CAD build for the part. Positions are in the model's coordinates, mm. A direction names the side the tool comes from. Round coordinates to 2 decimals unless told otherwise and drop trailing zeros. Write each loop counter-clockwise with the first axis right and the second up, starting at its lowest first coordinate (ties: lowest second). Pieces come first, ordered by that corner, then holes. Notation, with made-up numbers: (69, 35) - (95, 35) arc R20 ccw to (95, 65) - close; hole circle Ø2 at (-1, -36). An arc over 180 degrees is marked (long way). Use one line per item in the form item = value. Start each with the question number.
Item 1: Drill centre lines: L1, parallel to Z at x = -10.68, y = 13.55; L2, parallel to Y at x = 2, z = -3; L3, parallel to X at y = 9.5, z = 3.25. Where is each one in solid material? Low to high.
Item 2: Pull direction X, two halves, no side cores. Call faces 1 (the cylindrical face through (1.56, 7.23, 4.96)), 2 (the flat face through (6, 6, 0)), 3 (the flat face through (-1, 15.66, 0)): +X half, -X half, draft (parallel to the pull), parting line (faces both ways), or undercut.
Item 3: Tool access for faces 4 (the flat face through (0, 14.66, 0)), 5 (the flat face through (-2, 13, 7)), 6 (the flat face through (-4, 13, -7)), 7 (the cylindrical face through (-11.59, 13.05, -6.81)), 8 (the cylindrical face through (4.748, 15.098, 0.089)): list every direction of +Z, -Z, +X, -X, +Y, -Y with a clear straight run to the whole face (end or side of a thin tool).
Item 4: Pin check, flat tips, straight feed: pin 1 (4 mm diameter, centred on x = -8.5, z = -3.5, fed in from -Y); pin 2 (4 mm diameter, centred on x = -10.68, z = -8, fed in from +Y); pin 3 (4 mm diameter, centred on y = 5, z = -6, fed in from -X); pin 4 (2 mm diameter, centred on x = -7, y = 12, fed in from -Z). Stop position of each tip, or through.
Item 5: Band-saw the part on A-A, the plane z = -8. List the corners of the cut face in (x, y).
Item 6: Band-saw the part on D-D, the plane z = 8. List the corners of the cut face in (x, y).
Item 7: Band-saw the part on B-B, the plane x = -10.68. List the corners of the cut face in (y, z).
Item 8: Band-saw the part on C-C, the plane y = 1.75. List the corners of the cut face in (x, z).
from build123d import *
from build123d.topology import SkipClean

# Parameters (mm, degrees)
SKETCH1_R           = 7
SKETCH1_R_2         = 5.2
BOSS_EXTRUDE1_DEPTH = 15.66
BOSS_EXTRUDE2_START = -3.6
SKETCH2_W           = 6
SKETCH2_H           = 4
BOSS_EXTRUDE2_DEPTH = 3.6
CUT_EXTRUDE2_START  = -1.6
SKETCH2_3_W         = 6
SKETCH2_3_H         = 4
CUT_EXTRUDE2_DEPTH  = 1.6
SKETCH4_R           = 1.5
CUT_EXTRUDE1_DEPTH  = 10
FILLET7_R           = 3
BOSS_EXTRUDE3_START = -1
SKETCH5_R           = 5.2
BOSS_EXTRUDE3_DEPTH = 1
CUT_EXTRUDE3_DEPTH  = 15.66
FILLET8_R           = 3


with BuildPart() as part:
    # Sketch1 → Boss-Extrude1 (new body)
    with BuildSketch(Plane(origin=(0, 0, 0), x_dir=(1, 0, 0), z_dir=(0, 1, 0))):
        with Locations(Location((0, 0, 0), (0, 0, 270))):
            Circle(SKETCH1_R)
        with Locations(Location((0, 0, 0), (0, 0, 270))):
            Circle(SKETCH1_R_2, mode=Mode.SUBTRACT)
    extrude(amount=BOSS_EXTRUDE1_DEPTH)

    # Sketch2 → Boss-Extrude2 (add)
    with BuildSketch(Plane(origin=(0, 15.66, 0), x_dir=(1, 0, 0), z_dir=(0, 1, 0)).offset(BOSS_EXTRUDE2_START)):
        with Locations((-10.67, -9)):
            Rectangle(SKETCH2_W, SKETCH2_H)
        with BuildLine():
            ThreePointArc((0, -7), (-7, 0), (0, 7))
            Line((0, 7), (-7.67, 7))
            Line((-7.67, 7), (-13.67, 7))
            Line((-13.67, 7), (-13.67, -7))
            Line((-13.67, -7), (-7.67, -7))
            Line((-7.67, -7), (0, -7))
        make_face()
        with Locations((-10.67, 9)):
            Rectangle(SKETCH2_W, SKETCH2_H)
    extrude(amount=BOSS_EXTRUDE2_DEPTH)

    # Sketch2<3> → Cut-Extrude2 (cut)
    with SkipClean():  # the faces are left unmerged after this step: merging them gives an invalid solid
        with BuildSketch(Plane(origin=(0, 15.66, 0), x_dir=(1, 0, 0), z_dir=(0, 1, 0)).offset(CUT_EXTRUDE2_START)):
            with BuildLine():
                ThreePointArc((0, -7), (-7, 0), (0, 7))
                Line((0, 7), (-7.67, 7))
                Line((-7.67, 7), (-13.67, 7))
                Line((-13.67, 7), (-13.67, -7))
                Line((-13.67, -7), (-7.67, -7))
                Line((-7.67, -7), (0, -7))
            make_face()
            with Locations((-10.67, 9)):
                Rectangle(SKETCH2_3_W, SKETCH2_3_H)
            with Locations((-10.67, -9)):
                Rectangle(SKETCH2_3_W, SKETCH2_3_H)
        extrude(amount=CUT_EXTRUDE2_DEPTH, mode=Mode.SUBTRACT)

    # Sketch4 → Cut-Extrude1 (cut)
    with SkipClean():  # the faces are left unmerged after this step: merging them gives an invalid solid
        with BuildSketch(Plane.XZ.offset(-12.06)):
            with Locations(Location((-10.68, -8, 0), (0, 0, 270))):
                Circle(SKETCH4_R)
            with Locations(Location((-10.68, 8, 0), (0, 0, 270))):
                Circle(SKETCH4_R)
        extrude(amount=-CUT_EXTRUDE1_DEPTH, mode=Mode.SUBTRACT)

    # Fillet7
    fillet7_edges = [part.edges().sort_by_distance(p)[0] for p in [
        (-7.67, 13.06, 7),
    ]]
    fillet(fillet7_edges, radius=FILLET7_R)

    # Sketch5 → Boss-Extrude3 (add)
    with SkipClean():  # the faces are left unmerged after this step: merging them gives an invalid solid
        with BuildSketch(Plane(origin=(0, 15.66, 0), x_dir=(1, 0, 0), z_dir=(0, 1, 0)).offset(BOSS_EXTRUDE3_START)):
            with Locations(Location((0, 0, 0), (0, 0, 270))):
                Circle(SKETCH5_R)
        extrude(amount=BOSS_EXTRUDE3_DEPTH)

    # Sketch6 → Cut-Extrude3 (cut)
    with BuildSketch(Plane.XZ):
        with BuildLine():
            Line((6, -3.605551275), (6, 3.605551275))
            ThreePointArc((6, 3.605551275), (7, 0), (6, -3.605551275))
        make_face()
    extrude(amount=-CUT_EXTRUDE3_DEPTH, mode=Mode.SUBTRACT)

    # Fillet8
    fillet8_edges = [part.edges().sort_by_distance(p)[0] for p in [
        (6, 15.66, 0),
    ]]
    fillet(fillet8_edges, radius=FILLET8_R)


solid = part.part
Determined:
q1.L1 = -11 to -9.5, -6.5 to 6.5, 9.5 to 11
q1.L2 = 14.66 to 15.66
q1.L3 = -6.2 to -4.06, 4.06 to 6
q2.face_1 = undercut
q2.face_2 = +X half
q2.face_3 = draft
q3.face_4 = -Y
q3.face_5 = +Z, +X, +Y, -Y
q3.face_6 = -Z, +X, +Y, -Y
q3.face_7 = +Y, -Y
q3.face_8 = +Z, -Z, +X, +Y
q4.pin_1 = 12.06
q4.pin_2 = 14.06
q4.pin_3 = -5.74
q4.pin_4 = -11
q5.outline = (-13.67, 12.06) - (-12.18, 12.06) - (-12.18, 14.06) - (-13.67, 14.06) - close; (-9.18, 12.06) - (-7.67, 12.06) - (-7.67, 14.06) - (-9.18, 14.06) - close
q6.outline = (-13.67, 12.06) - (-12.18, 12.06) - (-12.18, 14.06) - (-13.67, 14.06) - close; (-9.18, 12.06) - (-6.91, 12.06) - (-6.91, 14.06) - (-9.18, 14.06) - close
q7.outline = (12.06, -11) - (14.06, -11) - (14.06, -9.5) - (12.06, -9.5) - close; (12.06, -6.5) - (14.06, -6.5) - (14.06, 6.5) - (12.06, 6.5) - close; (12.06, 9.5) - (14.06, 9.5) - (14.06, 11) - (12.06, 11) - close
q8.outline = (6, -3.61) - (6, 3.61) arc R7 ccw (long way) to start; hole circle Ø10.4 at (0, 0)
